Source: CAD feature listing. Evaluate the final solid. Frame: model axes, mm. Coordinates: 2 decimals unless noted, no trailing zeros. Order: outer loops, then holes, each group sorted by start corner. A loop starts at its lowest first (then second) coordinate and runs counter-clockwise, first axis right, second up.
Item 1: Contact query for flat-ended pins moving along their axis: P1, Ø3, axis at y = 6.5, z = -71, coming from the -X side; P2, Ø10, axis at x = -1.5, z = -93, coming from the -Y side; P3, Ø1.5, axis at x = -4, z = -51.5, coming from the +Y side. Output: stop coordinate, or through.
Item 2: Section B-B on y = -7. Return the cut outline in (x, z), then the cut area to 3 significant figures.
Item 3: Section C-C on z = -58. Return the cut outline in (x, y) (1 decimal).
Item 4: Section D-D on x = 7.25. Return the cut outline in (y, z).
Item 5: Ray query, line 1 (Z direction, x = -6, y = -6.5); line 2 (Y direction, x = -0.5, z = -36.5); line 3 (X direction, y = -3.5, z = -83.5). Return the intervals inside material, ascending.
from build123d import *

# Parameters (mm, degrees)
SKETCH1_R                = 9.525
BOSS_EXTRUDE1_DEPTH      = 6.35
SKETCH2_R                = 4.7625
BOSS_EXTRUDE2_DEPTH      = 127
BOSS_EXTRUDE3_DEPTH      = 1.27
BOSS_EXTRUDE3_DEPTH_BACK = 1.27


with BuildPart() as part:
    # Sketch1 → Boss-Extrude1 (new body)
    with BuildSketch(Plane.XY):
        Circle(SKETCH1_R)
    extrude(amount=BOSS_EXTRUDE1_DEPTH)

    # Sketch2 → Boss-Extrude2 (add)
    with BuildSketch(Plane(origin=(0, 0, 0), x_dir=(-1, 0, 0), z_dir=(0, 0, -1))):
        Circle(SKETCH2_R)
    extrude(amount=BOSS_EXTRUDE2_DEPTH)

    # Sketch3 → Boss-Extrude3 (add, two sides: drawn at the far end of the back side and taken through both)
    with BuildSketch(Plane(origin=(0, 0, 0), x_dir=(0, 0, -1), z_dir=(1, 0, 0)).offset(-BOSS_EXTRUDE3_DEPTH_BACK)):
        with BuildLine():
            Line((44.196, -4.7625), (44.196, 4.7625))
            Line((44.196, 4.7625), (44.196, 8.1915))
            ThreePointArc((44.196, 8.1915), (69.653798614, 7.333275757), (94.996, 4.7625))
            Line((94.996, 4.7625), (94.996, -4.7625))
            ThreePointArc((94.996, -4.7625), (69.653798614, -7.333275757), (44.196, -8.1915))
            Line((44.196, -8.1915), (44.196, -4.7625))
        make_face()
    extrude(amount=BOSS_EXTRUDE3_DEPTH + BOSS_EXTRUDE3_DEPTH_BACK)


solid = part.part
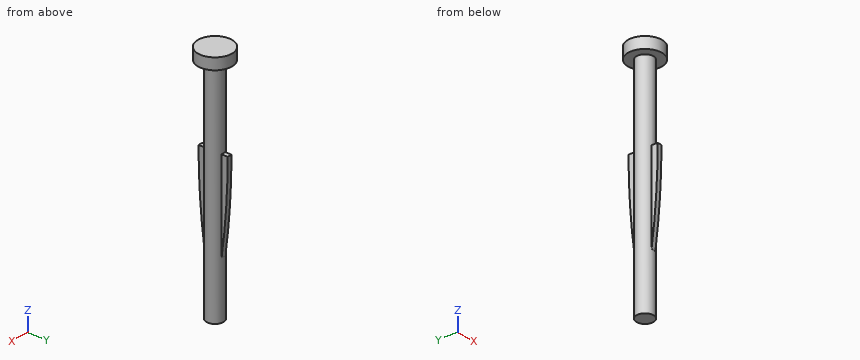
Answer list:
1. P1: stops at x = -1.27
1. P2: stops at y = -5.64
1. P3: stops at y = 3.48
2. outline: (-6.46, 0) - (6.46, 0) - (6.46, 6.35) - (-6.46, 6.35) - close; (-1.27, -74.19) - (1.27, -74.19) - (1.27, -44.2) - (-1.27, -44.2) - close
2. area: 158 mm2
3. outline: (-1.3, -7.9) - (1.3, -7.9) - (1.3, -4.6) arc R4.8 ccw to (1.3, 4.6) - (1.3, 7.9) - (-1.3, 7.9) - (-1.3, 4.6) arc R4.8 ccw to (-1.3, -4.6) - close
4. outline: (-6.18, 0) - (6.18, 0) - (6.18, 6.35) - (-6.18, 6.35) - close
5. line 1: z = 0 to 6.35
5. line 2: y = -4.74 to 4.74
5. line 3: x = -3.23 to 3.23
